```python
from build123d import *

# Parameters (mm, degrees)
EXTRUDE_1_DEPTH      = 43
EXTRUDE_1_DEPTH_BACK = 43
CUT_EXTRUDE_1_DEPTH  = 4
SKETCH_5_R           = 2.5
CUT_EXTRUDE_2_DEPTH  = 4
SKETCH_14_W          = 8.9
SKETCH_14_H          = 11
CUT_EXTRUDE_3_DEPTH  = 1.6
SKETCH_15_W          = 8.9
SKETCH_15_H          = 11
CUT_EXTRUDE_4_DEPTH  = 1.6
SKETCH_16_R          = 10
SKETCH_16_R_2        = 4
CUT_EXTRUDE_5_DEPTH  = 1.5
SKETCH_17_R          = 10
SKETCH_17_R_2        = 4
CUT_EXTRUDE_6_DEPTH  = 1.5
SKETCH_20_R          = 10
CUT_EXTRUDE_7_DEPTH  = 1.5
SKETCH_21_R          = 10
CUT_EXTRUDE_8_DEPTH  = 1.5


with BuildPart() as part:
    # Sketch 1 → Extrude 1 (new body, two sides)
    with BuildSketch(Plane.XY) as extrude_1_sk:
        with BuildLine():
            Line((-31, -30), (-16.5, -30))
            Line((-16.5, -30), (-16.5, -25))
            Line((-16.5, -25), (-7.6, -25))
            Line((-7.6, -25), (-7.6, -35.7))
            Line((-7.6, -35.7), (7.6, -35.7))
            Line((7.6, -35.7), (7.6, -25))
            Line((7.6, -25), (16.5, -25))
            Line((16.5, -25), (16.5, -30))
            Line((16.5, -30), (31, -30))
            Line((31, -30), (31, -7.5))
            Line((31, -7.5), (30.022875656, -7.5))
            ThreePointArc((30.022875656, -7.5), (26.7, -6), (30.022875656, -4.5))
            Line((30.022875656, -4.5), (31, -4.5))
            Line((31, -4.5), (31, 0))
            Line((31, 0), (9, 0))
            Line((9, 0), (8.7, -0.3))
            Line((8.7, -0.3), (-8.7, -0.3))
            Line((-8.7, -0.3), (-9, 0))
            Line((-9, 0), (-31, 0))
            Line((-31, 0), (-31, -4.5))
            Line((-31, -4.5), (-30.022875656, -4.5))
            ThreePointArc((-30.022875656, -4.5), (-26.7, -6), (-30.022875656, -7.5))
            Line((-30.022875656, -7.5), (-31, -7.5))
            Line((-31, -7.5), (-31, -30))
        make_face()
    extrude(amount=EXTRUDE_1_DEPTH)
    extrude(extrude_1_sk.sketch, amount=-EXTRUDE_1_DEPTH_BACK)

    # Sketch 2 → Cut-Revolve 1 (revolve, cut)
    with BuildSketch(Plane(origin=(0, 0, 0), x_dir=(0, 0, -1), z_dir=(1, 0, 0))):
        Polygon((19, -0.3), (22, -0.3), (21.4585, -0.8415), (21.4585, -15.3), (21.6, -15.3), (21.6, -25), (24, -25), (24, -35.7), (19, -35.7), align=None)
    revolve(axis=Axis((0, -35.7, -19), (0, 1, 0)), mode=Mode.SUBTRACT)

    # Sketch 3 → Cut-Revolve 2 (revolve, cut)
    with BuildSketch(Plane(origin=(0, 0, 0), x_dir=(0, 0, -1), z_dir=(1, 0, 0))):
        Polygon((-19, -0.3), (-16, -0.3), (-16.5415, -0.8415), (-16.5415, -15.3), (-16.4, -15.3), (-16.4, -25), (-14, -25), (-14, -35.7), (-19, -35.7), align=None)
    revolve(axis=Axis((0, -35.7, 19), (0, 1, 0)), mode=Mode.SUBTRACT)

    # Sketch 4 → Cut-Extrude 1 (cut)
    with BuildSketch(Plane(origin=(0, -0.3, 0), x_dir=(1, 0, 0), z_dir=(0, 1, 0))):
        with BuildLine():
            Line((-2.5, 37.5), (-2.5, 36.5))
            ThreePointArc((-2.5, 36.5), (0, 34), (2.5, 36.5))
            Line((2.5, 36.5), (2.5, 37.5))
            ThreePointArc((2.5, 37.5), (0, 40), (-2.5, 37.5))
        make_face()
    extrude(amount=-CUT_EXTRUDE_1_DEPTH, mode=Mode.SUBTRACT)

    # Sketch 5 → Cut-Extrude 2 (cut)
    with BuildSketch(Plane(origin=(0, -0.3, 0), x_dir=(1, 0, 0), z_dir=(0, 1, 0))):
        with Locations((0, -37)):
            Circle(SKETCH_5_R)
    extrude(amount=-CUT_EXTRUDE_2_DEPTH, mode=Mode.SUBTRACT)

    # Sketch 6 → Cut-Revolve 3 (revolve, cut)
    with BuildSketch(Plane(origin=(0, -25, 0), x_dir=(1, 0, 0), z_dir=(0, 1, 0))):
        Polygon((31, 28), (31, 25), (30.4585, 25.5415), (25, 25.5415), (25, 28), align=None)
    revolve(axis=Axis((25, -25, -28), (1, 0, 0)), mode=Mode.SUBTRACT)

    # Sketch 7 → Cut-Revolve 4 (revolve, cut)
    with BuildSketch(Plane(origin=(0, -25, 0), x_dir=(1, 0, 0), z_dir=(0, 1, 0))):
        Polygon((31, -28), (31, -31), (30.4585, -30.4585), (25, -30.4585), (25, -28), align=None)
    revolve(axis=Axis((25, -25, 28), (1, 0, 0)), mode=Mode.SUBTRACT)

    # Sketch 8 → Cut-Revolve 5 (revolve, cut)
    with BuildSketch(Plane(origin=(0, -25, 0), x_dir=(1, 0, 0), z_dir=(0, 1, 0))):
        Polygon((-25, 28), (-25, 25.5415), (-30.4585, 25.5415), (-31, 25), (-31, 28), align=None)
    revolve(axis=Axis((-31, -25, -28), (1, 0, 0)), mode=Mode.SUBTRACT)

    # Sketch 9 → Cut-Revolve 6 (revolve, cut)
    with BuildSketch(Plane(origin=(0, -25, 0), x_dir=(1, 0, 0), z_dir=(0, 1, 0))):
        Polygon((-25, -28), (-25, -30.4585), (-30.4585, -30.4585), (-31, -31), (-31, -28), align=None)
    revolve(axis=Axis((-31, -25, 28), (1, 0, 0)), mode=Mode.SUBTRACT)

    # Sketch 10 → Cut-Revolve 7 (revolve, cut)
    with BuildSketch(Plane(origin=(26, 0, 0), x_dir=(0, 0, -1), z_dir=(1, 0, 0))):
        Polygon((20, -30), (17, -30), (17.5415, -29.4585), (17.5415, -24), (20, -24), align=None)
    revolve(axis=Axis((26, -24, -20), (0, -1, 0)), mode=Mode.SUBTRACT)

    # Sketch 11 → Cut-Revolve 8 (revolve, cut)
    with BuildSketch(Plane(origin=(-26, 0, 0), x_dir=(0, 0, -1), z_dir=(1, 0, 0))):
        Polygon((-20, -30), (-23, -30), (-22.4585, -29.4585), (-22.4585, -24), (-20, -24), align=None)
    revolve(axis=Axis((-26, -24, 20), (0, -1, 0)), mode=Mode.SUBTRACT)

    # Sketch 12 → Cut-Revolve 9 (revolve, cut)
    with BuildSketch(Plane(origin=(-26, 0, 0), x_dir=(0, 0, -1), z_dir=(1, 0, 0))):
        Polygon((20, -30), (17, -30), (17.5415, -29.4585), (17.5415, -24), (20, -24), align=None)
    revolve(axis=Axis((-26, -24, -20), (0, -1, 0)), mode=Mode.SUBTRACT)

    # Sketch 13 → Cut-Revolve 10 (revolve, cut)
    with BuildSketch(Plane(origin=(26, 0, 0), x_dir=(0, 0, -1), z_dir=(1, 0, 0))):
        Polygon((-20, -30), (-23, -30), (-22.4585, -29.4585), (-22.4585, -24), (-20, -24), align=None)
    revolve(axis=Axis((26, -24, 20), (0, -1, 0)), mode=Mode.SUBTRACT)

    # Sketch 14 → Cut-Extrude 3 (cut)
    with BuildSketch(Plane(origin=(0, -25, 0), x_dir=(1, 0, 0), z_dir=(0, 1, 0))):
        with Locations((-12.05, -14.5)):
            Rectangle(SKETCH_14_W, SKETCH_14_H)
    extrude(amount=CUT_EXTRUDE_3_DEPTH, mode=Mode.SUBTRACT)

    # Sketch 15 → Cut-Extrude 4 (cut)
    with BuildSketch(Plane(origin=(0, -25, 0), x_dir=(1, 0, 0), z_dir=(0, 1, 0))):
        with Locations((12.05, 14.5)):
            Rectangle(SKETCH_15_W, SKETCH_15_H)
    extrude(amount=CUT_EXTRUDE_4_DEPTH, mode=Mode.SUBTRACT)

    # Sketch 16 → Cut-Extrude 5 (cut)
    with BuildSketch(Plane.XY.offset(43)):
        with Locations((16.5, -13)):
            Circle(SKETCH_16_R)
        with Locations((16.5, -13)):
            Circle(SKETCH_16_R_2, mode=Mode.SUBTRACT)
    extrude(amount=-CUT_EXTRUDE_5_DEPTH, mode=Mode.SUBTRACT)

    # Sketch 17 → Cut-Extrude 6 (cut)
    with BuildSketch(Plane.XY.offset(43)):
        with Locations((-16.5, -13)):
            Circle(SKETCH_17_R)
        with Locations((-16.5, -13)):
            Circle(SKETCH_17_R_2, mode=Mode.SUBTRACT)
    extrude(amount=-CUT_EXTRUDE_6_DEPTH, mode=Mode.SUBTRACT)

    # Sketch 18 → Cut-Revolve 11 (revolve, cut)
    with BuildSketch(Plane(origin=(0, -13, 0), x_dir=(1, 0, 0), z_dir=(0, 1, 0))):
        Polygon((16.5, -43), (14, -43), (14.433, -42.567), (14.433, -38), (16.5, -38), align=None)
    revolve(axis=Axis((16.5, -13, 38), (0, 0, 1)), mode=Mode.SUBTRACT)

    # Sketch 19 → Cut-Revolve 12 (revolve, cut)
    with BuildSketch(Plane(origin=(0, -13, 0), x_dir=(1, 0, 0), z_dir=(0, 1, 0))):
        Polygon((-16.5, -43), (-19, -43), (-18.567, -42.567), (-18.567, -38), (-16.5, -38), align=None)
    revolve(axis=Axis((-16.5, -13, 38), (0, 0, 1)), mode=Mode.SUBTRACT)

    # Sketch 20 → Cut-Extrude 7 (cut)
    with BuildSketch(Plane.XY.offset(-43)):
        with Locations((16.5, -13)):
            Circle(SKETCH_20_R)
    extrude(amount=CUT_EXTRUDE_7_DEPTH, mode=Mode.SUBTRACT)

    # Sketch 21 → Cut-Extrude 8 (cut)
    with BuildSketch(Plane.XY.offset(-43)):
        with Locations((-16.5, -13)):
            Circle(SKETCH_21_R)
    extrude(amount=CUT_EXTRUDE_8_DEPTH, mode=Mode.SUBTRACT)


solid = part.part
```
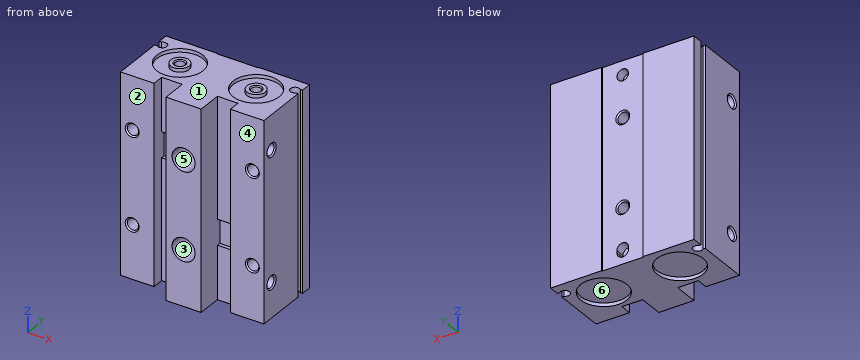
Design review of the part built by this model. Coordinates are the model's own, in mm. Face numbers are marked on the shaded views. A direction names the side the tool comes from. Coordinates: 2 decimals unless noted, no trailing zeros. Loops run counter-clockwise (first coordinate to the right, second up) from the corner with the lowest first, then second, coordinate; pieces in that order, holes last. Notation, with made-up numbers: (75, -7) -> (116, -7) arc R22 ccw to (116, 7) -> close; hole circle Ø3 at (55.25, -16). An arc over 180 degrees is marked (long way). Answer as a JSON object with one key per item and string values.
Q1. The part is to be moulded in two halves that separate along Z. For the marked faces 1, 2 and 3, say which applies: +Z half, -Z half, draft (parallel to the pull), parting line (faces both ways), or undercut.
Answer block:
{"face 1": "+Z half", "face 2": "draft", "face 3": "undercut"}
Q2. Take a section at B-B on y = -6. Give the boundary of the cut face in (x, z).
Answer block:
{"outline": "(-26.7, -43) -> (-23.64, -43) -> (-23.64, -41.5) -> (-9.36, -41.5) -> (-9.36, -43) -> (9.36, -43) -> (9.36, -41.5) -> (23.64, -41.5) -> (23.64, -43) -> (26.7, -43) -> (26.7, 43) -> (23.64, 43) -> (23.64, 41.5) -> (9.36, 41.5) -> (9.36, 43) -> (-9.36, 43) -> (-9.36, 41.5) -> (-23.64, 41.5) -> (-23.64, 43) -> (-26.7, 43) -> close; hole circle Ø4.92 at (0, -19); hole circle Ø4.92 at (0, 19)"}
Q3. To check wall thickness, follow L1, parallel to Z at x = -26, y = -28.1; L2, parallel to Z at x = 0, y = -21.75; L3, parallel to Z at x = -26, y = -25.15. State the ranges of each line that lie inside material, in increasing order.
Answer block:
{"L1": "z = -43 to -22.46, -17.54 to 17.54, 22.46 to 43", "L2": "z = -43 to -21.6, -16.4 to 16.4, 21.6 to 43", "L3": "z = -43 to -30.45, -25.55 to -22.46, -17.54 to 17.54, 22.46 to 25.55, 30.45 to 43"}
Q4. Tool access review of the marked faces 4, 5 and 6: name each direction out of +Z, -Z, +X, -X, +Y, -Y from which nothing blocks a thin tool from reaching the whole face with its end or side.
Answer block:
{"face 4": "+Z, -Z, +X, -Y", "face 5": "-Y", "face 6": "-Z"}
Q5. Clearance check with flat-ended pins moving along their axes: pin 1 Ø1.6 at (x, z) = (-1, -19) entering from -Y; pin 2 Ø11.5 at (x, z) = (0, 19) entering from +Y; pin 3 Ø4.5 at (x, z) = (26, -20) entering from -Y; pin 4 Ø7 at (x, z) = (-14, 16.5) entering from -Y. State where each tip first meets the part, or that it passes through.
Answer block:
{"pin 1": "passes through", "pin 2": "stops at y = -0.3", "pin 3": "stops at y = -24", "pin 4": "stops at y = -30"}
Q6. Take a section at C-C on y = -12. Give the number of separate pieces and of enclosed holes in the cut face, plus the area to 3 significant figures.
Answer block:
{"separate pieces": "1", "enclosed holes": "2", "area": "5,160 mm^2"}
Q7. Take a section at A-A on z = -1.5. Give the boundary of the cut face in (x, y).
Answer block:
{"outline": "(-31, -30) -> (-16.5, -30) -> (-16.5, -25) -> (-7.6, -25) -> (-7.6, -35.7) -> (7.6, -35.7) -> (7.6, -25) -> (16.5, -25) -> (16.5, -30) -> (31, -30) -> (31, -7.5) -> (30.02, -7.5) arc R2 cw (long way) to (30.02, -4.5) -> (31, -4.5) -> (31, 0) -> (9, 0) -> (8.7, -0.3) -> (-8.7, -0.3) -> (-9, 0) -> (-31, 0) -> (-31, -4.5) -> (-30.02, -4.5) arc R2 cw (long way) to (-30.02, -7.5) -> (-31, -7.5) -> close"}
